Verification items for this drawing (mm, ordinates from the low corner). A direction names the side the tool comes from. Round coordinates to 2 decimals unless told otherwise and drop trailing zeros. Loops run counter-clockwise (first coordinate to the right, second up) from the corner with the lowest first, then second, coordinate; pieces in that order, holes last. Notation, with made-up numbers: (-17.75, 74) -> (40.25, 74) arc R11 cw to (40.25, 84) -> close; hole circle Ø11 at (19, 6.25). An arc over 180 degrees is marked (long way). One line per question, with ' | ' between items.
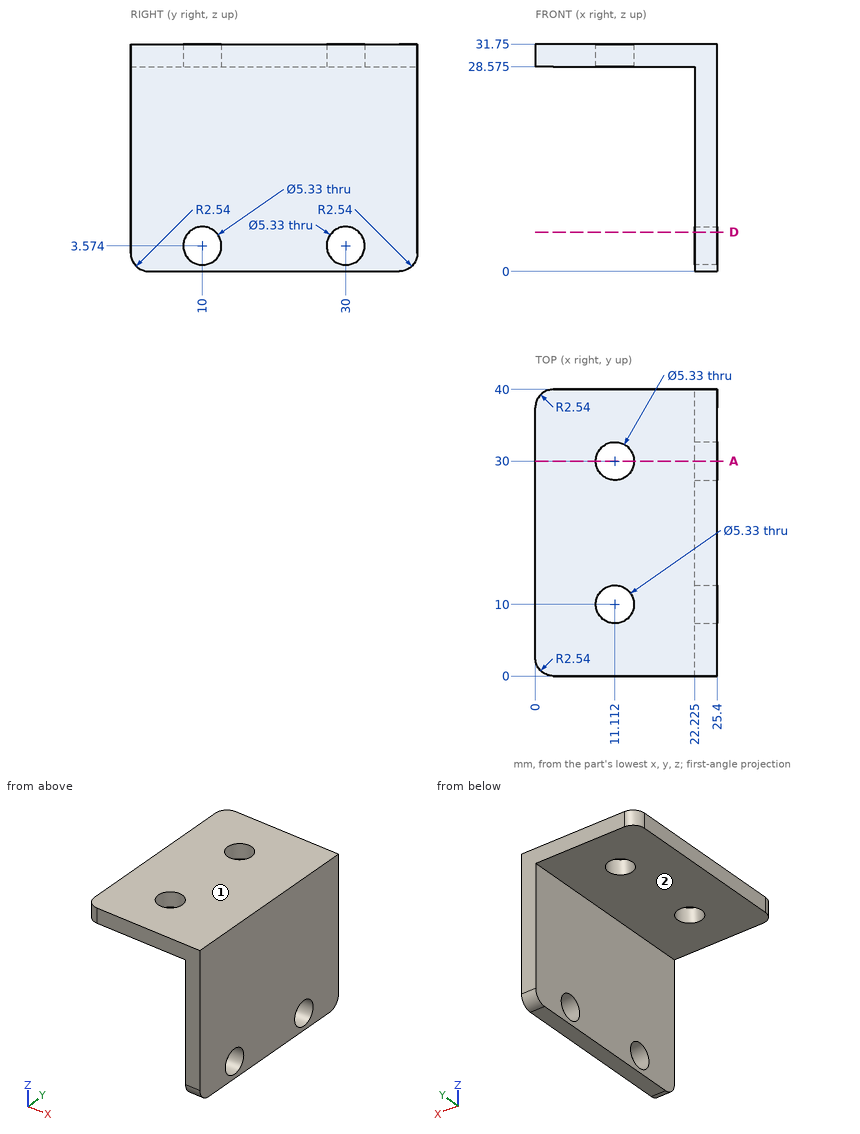
(1) Sectioned sample at A-A, the plane y = 30. Count the separate pieces of the cut face and the enclosed holes in it.
Answer:
separate pieces: 3 | enclosed holes: 0
(2) Scan line: probe 1 along X at (y, z) = (3.5, 9) (1 decimal). Record every from-to range of solid material in increasing order.
Answer:
probe 1: x = 22.2 to 25.4
(3) Sectioned sample at D-D, the plane z = 5.5. Record the cut outline in (x, y) (1 decimal), and give its area (3 significant figures).
Answer:
outline: (22.2, 0) -> (25.4, 0) -> (25.4, 8.2) -> (22.2, 8.2) -> close; (22.2, 11.8) -> (25.4, 11.8) -> (25.4, 28.2) -> (22.2, 28.2) -> close; (22.2, 31.8) -> (25.4, 31.8) -> (25.4, 40) -> (22.2, 40) -> close | area: 104 mm2
(4) Set-up check for the marked faces 1 and 2: record each of +Z, -Z, +X, -X, +Y, -Y from which the full face is reachable in a straight line by a thin tool's end or side.
Answer:
face 1: +Z, +X, -X, +Y, -Y | face 2: -Z, -X, +Y, -Y
(5) Go/stop test with flat-tipped pins: pin 1 (1 mm diameter, centred on x = 11.5, y = 10, fed in from +Z); pin 2 (6 mm diameter, centred on y = 30, z = 3.57, fed in from -X) (1 decimal); pin 3 (8.5 mm diameter, centred on x = 11.11, y = 10, fed in from -Z) (1 decimal); pin 4 (6 mm diameter, centred on x = 11.11, y = 30, fed in from +Z). Record where each tip stops, or that it passes through.
Answer:
pin 1: passes through | pin 2: stops at x = 22.2 | pin 3: stops at z = 28.6 | pin 4: stops at z = 31.75
